from build123d import *

# Parameters (mm, degrees)
SKETCH1_W             = 250
SKETCH1_H             = 130
BOSS_EXTRUDE1_DEPTH   = 3
SKETCH2_W             = 250
SKETCH2_H             = 1
BOSS_EXTRUDE2_DEPTH   = 25.5
SKETCH3_W             = 250
SKETCH3_H             = 1
BOSS_EXTRUDE3_DEPTH   = 22.5
SKETCH4_W             = 1
SKETCH4_H             = 128
BOSS_EXTRUDE4_DEPTH   = 22.5
SKETCH6_W             = 1
SKETCH6_H             = 14
BOSS_EXTRUDE5_DEPTH   = 22.5
SKETCH7_W             = 1
SKETCH7_H             = 14
BOSS_EXTRUDE6_DEPTH   = 22.5
SKETCH8_W             = 1
SKETCH8_H             = 13
BOSS_EXTRUDE7_DEPTH   = 21.5
SKETCH10_W            = 247
SKETCH10_H            = 1
BOSS_EXTRUDE8_DEPTH   = 21.5
SKETCH11_W            = 1
SKETCH11_H            = 127
BOSS_EXTRUDE9_DEPTH   = 21.5
SKETCH14_W            = 247
SKETCH14_H            = 1
BOSS_EXTRUDE10_DEPTH  = 21.5
SKETCH15_W            = 1
SKETCH15_H            = 12
BOSS_EXTRUDE11_DEPTH  = 21.5
FILLET1_R             = 1
SKETCH17_W            = 128
SKETCH17_H            = 1.2
BOSS_EXTRUDE12_DEPTH  = 10
SKETCH19_W            = 128
SKETCH19_H            = 1.2
BOSS_EXTRUDE13_DEPTH  = 10
SKETCH22_W            = 3
SKETCH22_H            = 10.8
BOSS_EXTRUDE14_DEPTH  = 21.5
SKETCH24_W            = 3
SKETCH24_H            = 10.8
BOSS_EXTRUDE15_DEPTH  = 21.5
SKETCH31_W            = 5
SKETCH31_H            = 10.8
BOSS_EXTRUDE16_DEPTH  = 4
SKETCH33_W            = 5
SKETCH33_H            = 10.8
BOSS_EXTRUDE18_DEPTH  = 4
SKETCH44_W            = 118
SKETCH44_H            = 4
BOSS_EXTRUDE28_DEPTH  = 21.5
SKETCH45_W            = 10
SKETCH45_H            = 12
BOSS_EXTRUDE29_DEPTH  = 21.5
SKETCH46_W            = 10
SKETCH46_H            = 8
BOSS_EXTRUDE30_DEPTH  = 21.5
SKETCH47_W            = 10
SKETCH47_H            = 10.8
BOSS_EXTRUDE31_DEPTH  = 21.5
SKETCH48_W            = 10
SKETCH48_H            = 10.8
BOSS_EXTRUDE32_DEPTH  = 21.5
SKETCH49_W            = 108
SKETCH49_H            = 4
BOSS_EXTRUDE33_DEPTH  = 21.5
SKETCH62_R            = 1.5
CASEMUNTHOLE001_DEPTH = 18
SKETCH63_R            = 1.5
CASEMUNTHOLE002_DEPTH = 18
SKETCH64_R            = 1.5
CASEMUNTHOLE003_DEPTH = 18
SKETCH65_R            = 1.5
CASEMUNTHOLE004_DEPTH = 18
SKETCH67_W            = 4
SKETCH67_H            = 102
BOSS_EXTRUDE35_DEPTH  = 21.5
SKETCH72_W            = 39
SKETCH72_H            = 9
CUT_EXTRUDE1_DEPTH    = 20
SKETCH73_W            = 13
SKETCH73_H            = 12.5
CUT_EXTRUDE2_DEPTH    = 20
SKETCH74_W            = 4
SKETCH74_H            = 2
CUT_EXTRUDE3_DEPTH    = 11.5
SKETCH75_W            = 4
SKETCH75_H            = 2
CUT_EXTRUDE4_DEPTH    = 11.5
FILLET2_R             = 2


with BuildPart() as part:
    # Sketch1 → Boss-Extrude1 (new body)
    with BuildSketch(Plane(origin=(0, 0, 0), x_dir=(1, 0, 0), z_dir=(0, 1, 0))):
        Rectangle(SKETCH1_W, SKETCH1_H)
    extrude(amount=BOSS_EXTRUDE1_DEPTH)

    # Sketch2 → Boss-Extrude2 (add)
    with BuildSketch(Plane(origin=(0, 0, 0), x_dir=(1, 0, 0), z_dir=(0, 1, 0))):
        with Locations((0, 64.5)):
            Rectangle(SKETCH2_W, SKETCH2_H)
    extrude(amount=BOSS_EXTRUDE2_DEPTH)

    # Sketch3 → Boss-Extrude3 (add)
    with BuildSketch(Plane(origin=(0, 3, 0), x_dir=(1, 0, 0), z_dir=(0, 1, 0))):
        with Locations((0, -64.5)):
            Rectangle(SKETCH3_W, SKETCH3_H)
    extrude(amount=BOSS_EXTRUDE3_DEPTH)

    # Sketch4 → Boss-Extrude4 (add)
    with BuildSketch(Plane(origin=(0, 3, 0), x_dir=(1, 0, 0), z_dir=(0, 1, 0))):
        with Locations((-124.5, 0)):
            Rectangle(SKETCH4_W, SKETCH4_H)
    extrude(amount=BOSS_EXTRUDE4_DEPTH)

    # Sketch6 → Boss-Extrude5 (add)
    with BuildSketch(Plane(origin=(0, 3, 0), x_dir=(1, 0, 0), z_dir=(0, 1, 0))):
        with Locations((124.5, -58)):
            Rectangle(SKETCH6_W, SKETCH6_H)
    extrude(amount=BOSS_EXTRUDE5_DEPTH)

    # Sketch7 → Boss-Extrude6 (add)
    with BuildSketch(Plane(origin=(0, 3, 0), x_dir=(1, 0, 0), z_dir=(0, 1, 0))):
        with Locations((124.5, 58)):
            Rectangle(SKETCH7_W, SKETCH7_H)
    extrude(amount=BOSS_EXTRUDE6_DEPTH)

    # Sketch8 → Boss-Extrude7 (add)
    with BuildSketch(Plane(origin=(0, 3, 0), x_dir=(1, 0, 0), z_dir=(0, 1, 0))):
        with Locations((123.5, 57.5)):
            Rectangle(SKETCH8_W, SKETCH8_H)
    extrude(amount=BOSS_EXTRUDE7_DEPTH)

    # Sketch10 → Boss-Extrude8 (add)
    with BuildSketch(Plane(origin=(0, 3, 0), x_dir=(1, 0, 0), z_dir=(0, 1, 0))):
        with Locations((-0.5, 63.5)):
            Rectangle(SKETCH10_W, SKETCH10_H)
    extrude(amount=BOSS_EXTRUDE8_DEPTH)

    # Sketch11 → Boss-Extrude9 (add)
    with BuildSketch(Plane(origin=(0, 3, 0), x_dir=(1, 0, 0), z_dir=(0, 1, 0))):
        with Locations((-123.5, -0.5)):
            Rectangle(SKETCH11_W, SKETCH11_H)
    extrude(amount=BOSS_EXTRUDE9_DEPTH)

    # Sketch14 → Boss-Extrude10 (add)
    with BuildSketch(Plane(origin=(0, 3, 0), x_dir=(1, 0, 0), z_dir=(0, 1, 0))):
        with Locations((0.5, -63.5)):
            Rectangle(SKETCH14_W, SKETCH14_H)
    extrude(amount=BOSS_EXTRUDE10_DEPTH)

    # Sketch15 → Boss-Extrude11 (add)
    with BuildSketch(Plane(origin=(0, 3, 0), x_dir=(1, 0, 0), z_dir=(0, 1, 0))):
        with Locations((123.5, -57)):
            Rectangle(SKETCH15_W, SKETCH15_H)
    extrude(amount=BOSS_EXTRUDE11_DEPTH)

    # Fillet1
    fillet1_edges = [part.edges().sort_by_distance(p)[0] for p in [
        (0, 0, 65),
        (-125, 0, 0),
        (0, 0, -65),
        (125, 0, 0),
        (125, 12.75, 65),
        (-125, 12.75, 65),
        (-125, 12.75, -65),
        (125, 12.75, -65),
    ]]
    fillet(fillet1_edges, radius=FILLET1_R)

    # Sketch17 → Boss-Extrude12 (add)
    with BuildSketch(Plane(origin=(0, 3, 0), x_dir=(1, 0, 0), z_dir=(0, 1, 0))):
        with Locations((59, 51.6)):
            Rectangle(SKETCH17_W, SKETCH17_H)
    extrude(amount=BOSS_EXTRUDE12_DEPTH)

    # Sketch19 → Boss-Extrude13 (add)
    with BuildSketch(Plane(origin=(0, 3, 0), x_dir=(1, 0, 0), z_dir=(0, 1, 0))):
        with Locations((59, -51.6)):
            Rectangle(SKETCH19_W, SKETCH19_H)
    extrude(amount=BOSS_EXTRUDE13_DEPTH)

    # Sketch22 → Boss-Extrude14 (add)
    with BuildSketch(Plane(origin=(0, 3, 0), x_dir=(1, 0, 0), z_dir=(0, 1, 0))):
        with Locations((-3.5, -57.6)):
            Rectangle(SKETCH22_W, SKETCH22_H)
    extrude(amount=BOSS_EXTRUDE14_DEPTH)

    # Sketch24 → Boss-Extrude15 (add)
    with BuildSketch(Plane(origin=(0, 3, 0), x_dir=(1, 0, 0), z_dir=(0, 1, 0))):
        with Locations((-3.5, 57.6)):
            Rectangle(SKETCH24_W, SKETCH24_H)
    extrude(amount=BOSS_EXTRUDE15_DEPTH)

    # Sketch31 → Boss-Extrude16 (add)
    with BuildSketch(Plane(origin=(0, 3, 0), x_dir=(1, 0, 0), z_dir=(0, 1, 0))):
        with Locations((72.5, -57.6)):
            Rectangle(SKETCH31_W, SKETCH31_H)
    extrude(amount=BOSS_EXTRUDE16_DEPTH)

    # Sketch33 → Boss-Extrude18 (add)
    with BuildSketch(Plane(origin=(0, 3, 0), x_dir=(1, 0, 0), z_dir=(0, 1, 0))):
        with Locations((72.5, 57.6)):
            Rectangle(SKETCH33_W, SKETCH33_H)
    extrude(amount=BOSS_EXTRUDE18_DEPTH)

    # Sketch44 → Boss-Extrude28 (add)
    with BuildSketch(Plane(origin=(0, 3, 0), x_dir=(1, 0, 0), z_dir=(0, 1, 0))):
        with Locations((-64, -53)):
            Rectangle(SKETCH44_W, SKETCH44_H)
    extrude(amount=BOSS_EXTRUDE28_DEPTH)

    # Sketch45 → Boss-Extrude29 (add)
    with BuildSketch(Plane(origin=(0, 3, 0), x_dir=(1, 0, 0), z_dir=(0, 1, 0))):
        with Locations((-118, 57)):
            Rectangle(SKETCH45_W, SKETCH45_H)
    extrude(amount=BOSS_EXTRUDE29_DEPTH)

    # Sketch46 → Boss-Extrude30 (add)
    with BuildSketch(Plane(origin=(0, 3, 0), x_dir=(1, 0, 0), z_dir=(0, 1, 0))):
        with Locations((-118, -59)):
            Rectangle(SKETCH46_W, SKETCH46_H)
    extrude(amount=BOSS_EXTRUDE30_DEPTH)

    # Sketch47 → Boss-Extrude31 (add)
    with BuildSketch(Plane(origin=(0, 3, 0), x_dir=(1, 0, 0), z_dir=(0, 1, 0))):
        with Locations((118, 57.6)):
            Rectangle(SKETCH47_W, SKETCH47_H)
    extrude(amount=BOSS_EXTRUDE31_DEPTH)

    # Sketch48 → Boss-Extrude32 (add)
    with BuildSketch(Plane(origin=(0, 3, 0), x_dir=(1, 0, 0), z_dir=(0, 1, 0))):
        with Locations((118, -57.6)):
            Rectangle(SKETCH48_W, SKETCH48_H)
    extrude(amount=BOSS_EXTRUDE32_DEPTH)

    # Sketch49 → Boss-Extrude33 (add)
    with BuildSketch(Plane(origin=(0, 3, 0), x_dir=(1, 0, 0), z_dir=(0, 1, 0))):
        with Locations((-59, 53)):
            Rectangle(SKETCH49_W, SKETCH49_H)
    extrude(amount=BOSS_EXTRUDE33_DEPTH)

    # Sketch62 → CaseMuntHole001 (cut)
    with BuildSketch(Plane(origin=(0, 24.5, 0), x_dir=(1, 0, 0), z_dir=(0, 1, 0))):
        with Locations((-119.5, 59.5)):
            Circle(SKETCH62_R)
    extrude(amount=-CASEMUNTHOLE001_DEPTH, mode=Mode.SUBTRACT)

    # Sketch63 → CaseMuntHole002 (cut)
    with BuildSketch(Plane(origin=(0, 24.5, 0), x_dir=(1, 0, 0), z_dir=(0, 1, 0))):
        with Locations((119.5, 59.5)):
            Circle(SKETCH63_R)
    extrude(amount=-CASEMUNTHOLE002_DEPTH, mode=Mode.SUBTRACT)

    # Sketch64 → CaseMuntHole003 (cut)
    with BuildSketch(Plane(origin=(0, 24.5, 0), x_dir=(1, 0, 0), z_dir=(0, 1, 0))):
        with Locations((119.5, -59.5)):
            Circle(SKETCH64_R)
    extrude(amount=-CASEMUNTHOLE003_DEPTH, mode=Mode.SUBTRACT)

    # Sketch65 → CaseMuntHole004 (cut)
    with BuildSketch(Plane(origin=(0, 24.5, 0), x_dir=(1, 0, 0), z_dir=(0, 1, 0))):
        with Locations((-119.5, -59.5)):
            Circle(SKETCH65_R)
    extrude(amount=-CASEMUNTHOLE004_DEPTH, mode=Mode.SUBTRACT)

    # Sketch67 → Boss-Extrude35 (add)
    with BuildSketch(Plane(origin=(0, 3, 0), x_dir=(1, 0, 0), z_dir=(0, 1, 0))):
        with Locations((-121, 0)):
            Rectangle(SKETCH67_W, SKETCH67_H)
    extrude(amount=BOSS_EXTRUDE35_DEPTH)

    # Sketch72 → Cut-Extrude1 (cut)
    with BuildSketch(Plane.ZY.offset(125)):
        with Locations((34, 21)):
            Rectangle(SKETCH72_W, SKETCH72_H)
    extrude(amount=-CUT_EXTRUDE1_DEPTH, mode=Mode.SUBTRACT)

    # Sketch73 → Cut-Extrude2 (cut)
    with BuildSketch(Plane.ZY.offset(125)):
        with Locations((8, 19.25)):
            Rectangle(SKETCH73_W, SKETCH73_H)
    extrude(amount=-CUT_EXTRUDE2_DEPTH, mode=Mode.SUBTRACT)

    # Sketch74 → Cut-Extrude3 (cut)
    with BuildSketch(Plane(origin=(0, 24.5, 0), x_dir=(1, 0, 0), z_dir=(0, 1, 0))):
        with Locations((-4, -52)):
            Rectangle(SKETCH74_W, SKETCH74_H)
    extrude(amount=-CUT_EXTRUDE3_DEPTH, mode=Mode.SUBTRACT)

    # Sketch75 → Cut-Extrude4 (cut)
    with BuildSketch(Plane(origin=(0, 24.5, 0), x_dir=(1, 0, 0), z_dir=(0, 1, 0))):
        with Locations((-4, 52)):
            Rectangle(SKETCH75_W, SKETCH75_H)
    extrude(amount=-CUT_EXTRUDE4_DEPTH, mode=Mode.SUBTRACT)

    # Fillet2
    fillet2_edges = [part.edges().sort_by_distance(p)[0] for p in [
        (113, 18.75, -52.2),
        (113, 18.75, 52.2),
    ]]
    fillet(fillet2_edges, radius=FILLET2_R)


solid = part.part
Check sheet for the modelled part. Datum: model origin and axes. Units: mm. A direction names the side the tool comes from. Give positions to 0.01 mm unless a question says otherwise; leave off trailing zeros. Write each loop counter-clockwise with the first axis right and the second up, starting at its lowest first coordinate (ties: lowest second). Pieces come first, ordered by that corner, then holes. Notation, with made-up numbers: (34.25, 21.25) -> (61.25, 21.25) arc R19 cw to (61.25, 26.25) -> close; hole circle Ø11 at (22, -13.75). An arc over 180 degrees is marked (long way). Write item = value, one per line.
Item 1: Sectioned sample at B-B on z = 41. Record the boundary of the cut face in (x, y), and give its area (3 significant figures).
Output:
outline = (-125, 1) arc R1 ccw to (-124, 0) -> (124, 0) arc R1 ccw to (125, 1) -> (125, 3) -> (-119, 3) -> (-119, 16.5) -> (-125, 16.5) -> close
area = 831 mm^2
Item 2: Sectioned sample at D-D on x = 28. Record the boundary of the cut face in (y, z).
Output:
outline = (0, -64) arc R1 ccw to (1, -65) -> (25.5, -65) -> (25.5, -64) -> (24.5, -64) -> (24.5, -63) -> (3, -63) -> (3, -52.2) -> (13, -52.2) -> (13, -51) -> (3, -51) -> (3, 51) -> (13, 51) -> (13, 52.2) -> (3, 52.2) -> (3, 63) -> (24.5, 63) -> (24.5, 64) -> (25.5, 64) -> (25.5, 65) -> (1, 65) arc R1 ccw to (0, 64) -> close
Item 3: Tool access check on faces 4 (the flat face through (-119, 11, 1)), 5 (the flat face through (94, 3, 58)), 6 (the flat face through (-120, 16.5, 38)). Record the directions out of +Z, -Z, +X, -X, +Y, -Y that give a thin tool (end or side, any length) a straight path to the whole face; none if there is none.
Output:
face_4 = +X, +Y
face_5 = +Y
face_6 = -X, +Y
Item 4: Sectioned sample at C-C on y = 19. Count the separate pieces of the cut face and the enclosed holes in it, and give its area (3 significant figures).
Output:
separate_pieces = 2
enclosed_holes = 6
area = 2,710 mm^2
Item 5: Sectioned sample at A-A on x = -73.5. Record the boundary of the cut face in (y, z), and give its area (3 significant figures).
Output:
outline = (0, -64) arc R1 ccw to (1, -65) -> (25.5, -65) -> (25.5, -64) -> (24.5, -64) -> (24.5, -63) -> (3, -63) -> (3, -55) -> (24.5, -55) -> (24.5, -51) -> (3, -51) -> (3, 51) -> (24.5, 51) -> (24.5, 55) -> (3, 55) -> (3, 63) -> (24.5, 63) -> (24.5, 64) -> (25.5, 64) -> (25.5, 65) -> (1, 65) arc R1 ccw to (0, 64) -> close
area = 650 mm^2
Item 6: Release check for a two-part mould opening along Z. For faces 1 (the flat face through (125, 1.4, 0.3)), 2 (the flat face through (-2, 13, 65)), 3 (the flat face through (-60, 14, -63)) record: +Z half, -Z half, draft (parallel to the pull), parting line (faces both ways), or undercut.
Output:
face_1 = draft
face_2 = +Z half
face_3 = undercut
Item 7: Gauge pin test, flat ends, axial feed: pin 1 (3.5 mm diameter, centred on x = -120, z = 60, fed in from +Y); pin 2 (12 mm diameter, centred on x = 42, z = -55.5, fed in from +Y); pin 3 (6 mm diameter, centred on x = -115, z = 33, fed in from +Y). Record the tip position at first contact, or that the pin passes through.
Output:
pin_1 = 24.5
pin_2 = 13
pin_3 = 3
Item 8: Scan lines: probe 1 along Z at (x, y) = (-119.5, 20.75); probe 2 along Z at (x, y) = (85, 7.5); probe 3 along X at (y, z) = (16.5, 59.5). Record each from-to range of solid material in increasing order. Write a range as from..to.
Output:
probe_1 = -65..-61, -58..1.5, 53.5..58, 61..65
probe_2 = -65..-63, -52.2..-51, 51..52.2, 63..65
probe_3 = -125..-121, -118..-113, -5..-2, 113..118, 121..125
